```python
from build123d import *

# Parameters (mm, degrees)
SKETCH1_R           = 8.5
SKETCH1_R_2         = 7.5
EXTRUDE_THIN1_DEPTH = 10
SKETCH2_R           = 13.024850754
BOSS_EXTRUDE1_DEPTH = 80
BOSS_EXTRUDE1_TAPER = 9
SCALE1_SCALE        = 10
SCALE2_SCALE        = 0.75


with BuildPart() as part:
    # Sketch1 → Extrude-Thin1 (new body)
    with BuildSketch(Plane.XY):
        Circle(SKETCH1_R)
        Circle(SKETCH1_R_2, mode=Mode.SUBTRACT)
    extrude(amount=EXTRUDE_THIN1_DEPTH)

    # Sketch2 → Boss-Extrude1 (add)
    with BuildSketch(Plane(origin=(0, 0, 0), x_dir=(-1, 0, 0), z_dir=(0, 0, -1))):
        Circle(SKETCH2_R)
    extrude(amount=BOSS_EXTRUDE1_DEPTH, taper=BOSS_EXTRUDE1_TAPER)


with BuildPart() as part_1:
    # Scale1: scaled about (0, 0, 0)
    add(part.part.scale(SCALE1_SCALE))


with BuildPart() as part_2:
    # Scale2: scaled about (0, 0, 0)
    add(part_1.part.scale(SCALE2_SCALE))


solid = part_2.part
```
Geometry: final body of the model. Coordinates: model frame, mm. A direction names the side the tool comes from. Round coordinates to 2 decimals unless told otherwise and drop trailing zeros. Order: outer loops, then holes, each group sorted by start corner. A loop starts at its lowest first (then second) coordinate and runs counter-clockwise, first axis right, second up. Notation, with made-up numbers: (10, -32) - (41, -32) arc R22 ccw to (41, 7) - close; hole circle Ø6 at (66.5, -12.5). An arc over 180 degrees is marked (long way). Use CSV: the item, a comma, the result in double quotes. Start each with the question number.
Q1. Section query B-B (z = -533). Return loops of the section in (x, y), and give its area (3 significant figures).
Q2. Mould query, pull axis X, two halves, no side actions, for faces 3 (the face through (-13.82, -62.234, 36.975)), 4 (the face through (-0.3, -56.4, 75)), 5 (the face through (-56.196, 2.473, 36.975)). Classes: +X half, -X half, draft (parallel to the pull), parting line (faces both ways), or undercut.
Q3. Material intervals for line 1 along X through (y, z) = (-2.5, 30); line 2 along Y through (x, z) = (0, 52); line 3 along Y through (x, z) = (8.5, -386.5), sorted ascending. Write a range as from..to.
Q4. Access query for faces 1 (the face through (10.73, -48.33, -304.2)), 2 (the face through (1, -64, 0)). Directions: +Z, -Z, +X, -X, +Y, -Y. A direction counts if a zero-diameter tool reaches every point of the face in a straight line with its end or side. Return the directions, or none.
Q5. First-contact query: pin 1 (1 mm diameter, centred on x = -25.5, z = -73.5, fed in from +Y); pin 2 (3 mm diameter, centred on x = 10, z = -269, fed in from -Y); pin 3 (8 mm diameter, centred on y = 59, z = -77, fed in from -X). Flat tips, straight axial feed; report the tip coordinate or a pass-through.
Q6. Section query A-A (z = -36.5). Return loops of the section in (x, y).
Result set:
1,outline,"circle Ø26.53 at (0, 0)"
1,area,"553 mm2"
2,face 3,"parting line"
2,face 4,"draft"
2,face 5,"undercut"
3,line 1,"x = -63.7..-56.19, 56.19..63.7"
3,line 2,"y = -63.75..-56.25, 56.25..63.75"
3,line 3,"y = -35.47..35.47"
4,face 1,"-Z"
4,face 2,"+Z"
5,pin 1,"stops at y = 82.35"
5,pin 2,"stops at y = -54.52"
5,pin 3,"stops at x = -65.55"
6,outline,"circle Ø183.81 at (0, 0)"
